Here's how the part is built. I have some questions about the finished solid (model axes, mm). A direction names the side the tool comes from. Give positions to 0.01 mm unless a question says otherwise; leave off trailing zeros. Write each loop counter-clockwise with the first axis right and the second up, starting at its lowest first coordinate (ties: lowest second). Pieces come first, ordered by that corner, then holes. Notation, with made-up numbers: (26, 78.5) - (38, 78.5) arc R28 cw to (38, 97.5) - close; hole circle Ø11 at (29.25, 8.5). An arc over 180 degrees is marked (long way). Use a Markdown table: item, result.
```python
from build123d import *

# Parameters (mm, degrees)
CROQUIS1_R              = 3.5
CROQUIS1_R_2            = 2.5
SALIENTE_EXTRUIR1_DEPTH = 3.7
SALIENTE_EXTRUIR2_DEPTH = 1


with BuildPart() as part:
    # Croquis1 → Saliente-Extruir1 (new body)
    with BuildSketch(Plane(origin=(0, 0, 0), x_dir=(1, 0, 0), z_dir=(0, 1, 0))):
        Circle(CROQUIS1_R)
        Circle(CROQUIS1_R_2, mode=Mode.SUBTRACT)
    extrude(amount=SALIENTE_EXTRUIR1_DEPTH)

    # Croquis2 → Saliente-Extruir2 (add)
    with BuildSketch(Plane(origin=(0, 3.7, 0), x_dir=(1, 0, 0), z_dir=(0, 1, 0))):
        with BuildLine():
            Line((-14.15, 1.85), (0, 3.5))
            Line((0, 3.5), (14.15, 1.85))
            ThreePointArc((14.15, 1.85), (16, 0), (14.15, -1.85))
            Line((14.15, -1.85), (0, -3.5))
            Line((0, -3.5), (-14.15, -1.85))
            ThreePointArc((-14.15, -1.85), (-16, 0), (-14.15, 1.85))
        make_face()
    extrude(amount=-SALIENTE_EXTRUIR2_DEPTH)


solid = part.part
```
Item 1: If we section it at B-B, the plane x = 0: Write out the boundary of the cut face in (y, z), plus the area to 3 significant figures.
Values:
| item | result |
|---|---|
| outline | (0, -3.5) - (3.7, -3.5) - (3.7, 3.5) - (0, 3.5) - (0, 2.5) - (2.7, 2.5) - (2.7, -2.5) - (0, -2.5) - close |
| area | 12.4 mm2 |
Item 2: If we section it at C-C, the plane z = 0: Write out the boundary of the cut face in (x, y), plus the area to 3 significant figures.
Values:
| item | result |
|---|---|
| outline | (-16, 2.7) - (-3.5, 2.7) - (-3.5, 0) - (-2.5, 0) - (-2.5, 2.7) - (2.5, 2.7) - (2.5, 0) - (3.5, 0) - (3.5, 2.7) - (16, 2.7) - (16, 3.7) - (-16, 3.7) - close |
| area | 37.4 mm2 |
Item 3: If we section it at A-A, the plane y = 3.1: Write out the boundary of the cut face in (x, z), plus the area to 3 significant figures.
Values:
| item | result |
|---|---|
| outline | (-14.15, -1.85) - (-0.81, -3.41) arc R3.5 ccw to (0.81, -3.41) - (14.15, -1.85) arc R1.85 ccw to (14.15, 1.85) - (0.81, 3.41) arc R3.5 ccw to (-0.81, 3.41) - (-14.15, 1.85) arc R1.85 ccw to start |
| area | 162 mm2 |
Item 4: I need wall thicknesses on line 1 along X through (y, z) = (1, 0); line 2 along X through (y, z) = (1.1, -1.25). Which ranges of each line are inside material? Lowest first, please. Write a range as [from, to].
Values:
| item | result |
|---|---|
| line 1 | x = [-3.5, -2.5], [2.5, 3.5] |
| line 2 | x = [-3.27, -2.17], [2.17, 3.27] |
Item 5: Will these pins go through, and if not, where does the flat tip stop? pin 1 Ø1 at (x, y) = (8.5, 2.5) entering from -Z; pin 2 Ø1.5 at (x, y) = (-3, 2) entering from -Z; pin 3 Ø4 at (x, z) = (0, 0) entering from -Y.
Values:
| item | result |
|---|---|
| pin 1 | stops at z = -2.56 |
| pin 2 | stops at z = -3.18 |
| pin 3 | stops at y = 2.7 |
Item 6: For faces 1 (the flat face through (0, 2.7, 0)), 2 (the flat face through (0, 3.7, 0)), which set-ups out of +Z, -Z, +X, -X, +Y, -Y let a thin tool reach every point of the face, with its end or its side?
Values:
| item | result |
|---|---|
| face 1 | -Y |
| face 2 | +Z, -Z, +X, -X, +Y |
Item 7: Thinking about a two-plate mould opening in Z: for faces 3 (the flat face through (7.571, 3.207, 2.617)), 4 (the cylindrical face through (-0.54, 1.33, 2.44)), 5 (the flat face through (9, 2.7, 0)), which applies, +Z half, -Z half, draft (parallel to the pull), parting line (faces both ways), or undercut?
Values:
| item | result |
|---|---|
| face 3 | +Z half |
| face 4 | undercut |
| face 5 | draft |
Item 8: If we section it at D-D, the plane y = 1.75: Write out the boundary of the cut face in (x, z).
Values:
| item | result |
|---|---|
| outline | circle Ø7 at (0, 0); hole circle Ø5 at (0, 0) |
